For this review, take the finished solid that the model builds, in its own axes (mm). Give positions to 0.01 mm unless a question says otherwise; leave off trailing zeros. Order: outer loops, then holes, each group sorted by start corner. A loop starts at its lowest first (then second) coordinate and runs counter-clockwise, first axis right, second up.
from build123d import *

# Parameters (mm, degrees)
SKETCH1_R                             = 7.5
SKETCH1_R_2                           = 27.5
F_125_IN_SHEET_DEPTH                  = 1.5875
FILLET1_R                             = 7
SKETCH2_R                             = 13
CUT_EXTRUDE1_DEPTH                    = 44.223370409
M4_CLEARANCE_HOLE1_D                  = 4.3
F_5_0_REAMED_OVER_FOR_SHOULDER_BOLT_D = 5


with BuildPart() as part:
    # Sketch1 → .125 in sheet (new, symmetric)
    with BuildSketch(Plane.XY):
        with Locations((22.980970389, 22.980970389)):
            Circle(SKETCH1_R)
        Circle(SKETCH1_R_2)
        with Locations((-22.980970389, 22.980970389)):
            Circle(SKETCH1_R)
        with Locations((-22.980970389, -22.980970389)):
            Circle(SKETCH1_R)
        with Locations((22.980970389, -22.980970389)):
            Circle(SKETCH1_R)
    extrude(amount=F_125_IN_SHEET_DEPTH, both=True)

    # Fillet1
    fillet1_edges = [part.edges().sort_by_distance(p)[0] for p in [
        (15.485317723, -22.725644876, 0),
        (-15.485317723, -22.725644876, 0),
        (-22.725644876, -15.485317723, 0),
        (-22.725644876, 15.485317723, 0),
        (-15.485317723, 22.725644876, 0),
        (15.485317723, 22.725644876, 0),
        (22.725644876, 15.485317723, 0),
        (22.725644876, -15.485317723, 0),
    ]]
    fillet(fillet1_edges, radius=FILLET1_R)

    # Sketch2 → Cut-Extrude1 (cut, through all)
    with BuildSketch(Plane.XY.offset(1.5875)):
        Circle(SKETCH2_R)
    extrude(amount=-CUT_EXTRUDE1_DEPTH, mode=Mode.SUBTRACT)

    # M4 Clearance Hole1 (through all)
    with Locations(Plane.XY.offset(1.5875)):
        with Locations((-12.374368671, 12.374368671), (12.374368671, 12.374368671), (12.374368671, -12.374368671), (-12.374368671, -12.374368671)):
            Hole(M4_CLEARANCE_HOLE1_D / 2)

    # Ø5.0 Reamed over for shoulder bolt (through all)
    with Locations(Plane.XY.offset(1.5875)):
        with Locations((-22.980970389, 22.980970389), (22.980970389, 22.980970389), (22.980970389, -22.980970389), (-22.980970389, -22.980970389)):
            Hole(F_5_0_REAMED_OVER_FOR_SHOULDER_BOLT_D / 2)


solid = part.part
1) To check wall thickness, follow line 1 (Y direction, x = 11.5, z = -0.7); line 2 (X direction, y = 24.5, z = 0.75); line 3 (X direction, y = 14, z = -0.75). State the ranges of each line that lie inside material, in increasing order.
Answer sheet:
line 1: y = -25.38 to -14.34, -10.41 to -6.06, 6.06 to 10.41, 14.34 to 25.38
line 2: x = -30.33 to -24.97, -21 to 21, 24.97 to 30.33
line 3: x = -25.68 to -13.78, -10.97 to 10.97, 13.78 to 25.68
2) Clearance check with flat-ended pins moving along their axes: pin 1 (2.5 mm diameter, centred on x = -12.37, y = -12.37, fed in from +Z); pin 2 (1.5 mm diameter, centred on x = -21.5, z = -0.5, fed in from +Y). State where each tip first meets the part, or that it passes through.
Answer sheet:
pin 1: passes through
pin 2: stops at y = 30.45
3) We need section C-C on z = 0.1. Count the separate pieces of the cut face and the enclosed holes in it, then the cut area to 3 significant figures.
Answer sheet:
separate pieces: 1
enclosed holes: 9
area: 2,410 mm2
4) Draft analysis for pull direction X (two halves, no side actions). For faces 1 (the face through (27.5, -0.1, 0)), 2 (the face through (-13.37, 10.47, -0.02)), 3 (the face through (13, -6, 1.588)), state which applies: +X half, -X half, draft (parallel to the pull), parting line (faces both ways), or undercut.
Answer sheet:
face 1: +X half
face 2: undercut
face 3: draft
5) We need section D-D on y = -19.5. Give the boundary of the cut face in (x, z), then the cut area to 3 significant figures.
Answer sheet:
outline: (-29.62, -1.59) - (29.62, -1.59) - (29.62, 1.59) - (-29.62, 1.59) - close
area: 188 mm2
6) We need section A-A on y = 0. Give the boundary of the cut face in (x, z).
Answer sheet:
outline: (-27.5, -1.59) - (-13, -1.59) - (-13, 1.59) - (-27.5, 1.59) - close; (13, -1.59) - (27.5, -1.59) - (27.5, 1.59) - (13, 1.59) - close
